Part model, mm, in its own coordinate system. Face numbers are marked on the shaded views. A direction names the side the tool comes from. Coordinates: 2 decimals unless noted, no trailing zeros. Order: outer loops, then holes, each group sorted by start corner. A loop starts at its lowest first (then second) coordinate and runs counter-clockwise, first axis right, second up.
1) Cut at A-A (z = 0). List the corners of the cut face in (x, y), and give its area (3 significant figures).
2) Cut at D-D (z = 7.5). List the corners of the cut face in (x, y), and give its area (3 significant figures).
3) Mould opens along Z. For the marked faces 3, 4, 5 and 6 say: +Z half, -Z half, draft (parallel to the pull), parting line (faces both ways), or undercut.
4) Cut at C-C (y = -15.75). List the corners of the cut face in (x, z).
5) Wall check: L1, parallel to Z at x = 0, y = -6; L2, parallel to Y at x = 4.5, z = -2; L3, parallel to X at y = -8, z = -11. Give the ranges that are in metal, low to high.
6) Cut at B-B (x = 0). List the corners of the cut face in (y, z), and give its area (3 significant figures).
7) Pin check, flat tips, straight feed: pin 1 Ø11 at (x, z) = (0.5, -4.5) entering from +Y; pin 2 Ø10 at (x, y) = (5.5, -17) entering from -Z; pin 3 Ø5 at (y, z) = (-6.5, 9.5) entering from -X. Stop position of each tip, or through.
8) Tool access for the marked faces 1 and 2: list every direction of +Z, -Z, +X, -X, +Y, -Y with a clear straight run to the whole face (end or side of a thin tool).
```python
from build123d import *

# Parameters (mm, degrees)
F0_R     = 15
F1_DEPTH = 24
F2_W     = 11
F2_H     = 3
F3_DEPTH = 15
F5_R     = 3.056512
F5_R_2   = 1.567652
F6_DEPTH = 10


with BuildPart() as f1:
    # F0 (on Front) → F1 (new body)
    with BuildSketch(Plane.XZ):
        Circle(F0_R)
        with BuildLine():
            ThreePointArc((2, -2.236068), (0, -3), (-2, -2.236068))
            Line((-2, -2.236068), (-2, 2.236068))
            ThreePointArc((-2, 2.236068), (0, 3), (2, 2.236068))
            Line((2, 2.236068), (2, -2.236068))
        make_face(mode=Mode.SUBTRACT)
    extrude(amount=F1_DEPTH)

    # F2 (on Top) → F3 (cut, symmetric)
    with BuildSketch(Plane.XY):
        with Locations((-5.5, -1.5)):
            Rectangle(F2_W, F2_H)
        with Locations((5.5, -1.5)):
            Rectangle(F2_W, F2_H)
    extrude(amount=F3_DEPTH, both=True, mode=Mode.SUBTRACT)

    # F5 (on offset) → F6 (join)
    with BuildSketch(Plane(origin=(0, -3, 0), x_dir=(-1, 0, 0), z_dir=(0, 1, 0))):
        Circle(F5_R)
        Circle(F5_R_2, mode=Mode.SUBTRACT)
    extrude(amount=-F6_DEPTH)


solid = f1.part
```
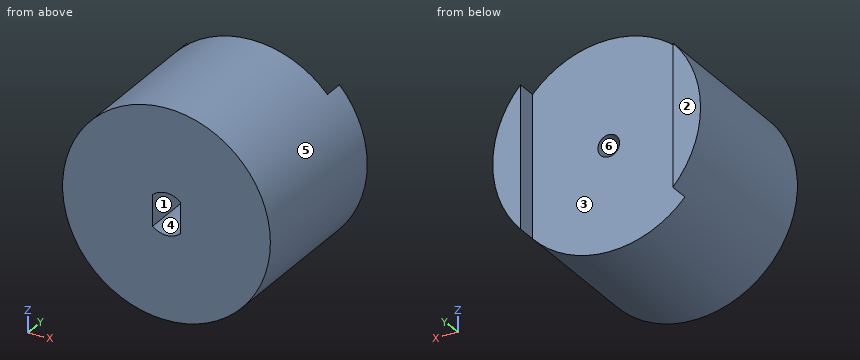
Geometry check:
1. outline: (-15, -24) - (-2, -24) - (-2, -13) - (-1.57, -13) - (-1.57, -3) - (-11, -3) - (-11, 0) - (-15, 0) - close; (1.57, -13) - (2, -13) - (2, -24) - (15, -24) - (15, 0) - (11, 0) - (11, -3) - (1.57, -3) - close
1. area: 579 mm2
2. outline: (-12.99, -24) - (12.99, -24) - (12.99, 0) - (11, 0) - (11, -3) - (-11, -3) - (-11, 0) - (-12.99, 0) - close
2. area: 558 mm2
3. face 3: draft
3. face 4: undercut
3. face 5: parting line
3. face 6: undercut
4. outline: circle Ø30 at (0, 0); hole (-2, -2.24) arc R3 ccw to (2, -2.24) - (2, 2.24) arc R3 ccw to (-2, 2.24) - close
5. L1: z = -15 to -1.57, 1.57 to 15
5. L2: y = -24 to -3
5. L3: x = -10.2 to 10.2
6. outline: (-24, -15) - (-3, -15) - (-3, -1.57) - (-13, -1.57) - (-13, -3) - (-24, -3) - close; (-24, 3) - (-13, 3) - (-13, 1.57) - (-3, 1.57) - (-3, 15) - (-24, 15) - close
6. area: 533 mm2
7. pin 1: stops at y = -3
7. pin 2: stops at z = -14.99
7. pin 3: stops at x = -13.27
8. face 1: -Y
8. face 2: +Z, -Z, +X, -X, +Y
